```python
from build123d import *

# Parameters (mm, degrees)
SKETCH6_R                = 15
SKETCH6_R_2              = 11
BOSS_EXTRUDE2_DEPTH      = 21.3
SKETCH4_W                = 19.7
SKETCH4_H                = 3
BOSS_EXTRUDE3_REACH      = 38.107
SKETCH9_W                = 21.3
SKETCH9_H                = 9.16515139
BOSS_EXTRUDE4_START      = 0.75
SKETCH10_R               = 15
SKETCH10_R_2             = 14.25
BOSS_EXTRUDE4_DEPTH      = 0.75
CHAMFER1_SIZE            = 0.5
CHAMFER1_OF_MIRROR1_SIZE = 0.5
BOSS_EXTRUDE6_DEPTH      = 21.3
SKETCH17_W               = 18.5
SKETCH17_H               = 23.6
CUT_EXTRUDE3_DEPTH       = 2
SKETCH14_R               = 11
CUT_EXTRUDE2_DEPTH       = 31.061936082
SKETCH18_W               = 32
SKETCH18_H               = 36
BOSS_EXTRUDE7_DEPTH      = 4
SKETCH19_W               = 28.2
SKETCH19_H               = 32.35
CUT_EXTRUDE4_DEPTH       = 2
SKETCH20_W               = 6
SKETCH20_H               = 16
SKETCH20_W_2             = 8
CUT_EXTRUDE5_DEPTH       = 1
SKETCH21_W               = 1.9
SKETCH21_H               = 16
SKETCH21_H_2             = 16.00994424
CUT_EXTRUDE6_DEPTH       = 0.5
SKETCH22_W               = 18.909915591
SKETCH22_H               = 1.825
CUT_EXTRUDE7_DEPTH       = 2
FILLET1_R                = 6
FILLET2_R                = 3


# Read off the part's stored shape, not the designer's step: Boss-Extrude6
with BuildPart() as part:
    # Sketch6 → Boss-Extrude2 (new body)
    with BuildSketch(Plane(origin=(0, 0, 0), x_dir=(0, 0, -1), z_dir=(1, 0, 0))):
        Circle(SKETCH6_R)
        Circle(SKETCH6_R_2, mode=Mode.SUBTRACT)
    extrude(amount=BOSS_EXTRUDE2_DEPTH)

    # Sketch4 → Cut-Revolve1 (revolve, cut)
    with BuildSketch(Plane.XY, mode=Mode.PRIVATE) as cut_revolve1_sk:
        with Locations((10.65, -13.5)):
            Rectangle(SKETCH4_W, SKETCH4_H)
    revolve(cut_revolve1_sk.sketch.rotate(Axis((-11.602577702, 0, 0), (1, 0, 0)), 270), axis=Axis((-11.602577702, 0, 0), (1, 0, 0)), mode=Mode.SUBTRACT)

    # Sketch9 → Boss-Extrude3 (add, up to next)
    with BuildSketch(Plane.XY.offset(-10), mode=Mode.PRIVATE) as boss_extrude3_sk1:
        with Locations((10.65, 0)):
            Rectangle(SKETCH9_W, SKETCH9_H)
    boss_extrude3_tool1 = extrude(boss_extrude3_sk1.sketch, amount=-BOSS_EXTRUDE3_REACH, mode=Mode.PRIVATE) - part.part
    add(boss_extrude3_tool1.solids().sort_by_distance((10.65, 0, -10))[0])

    # Sketch10 → Boss-Extrude4 (add)
    with BuildSketch(Plane.ZY.offset(-20.5).offset(BOSS_EXTRUDE4_START)):
        Circle(SKETCH10_R)
        Circle(SKETCH10_R_2, mode=Mode.SUBTRACT)
    boss_extrude4 = extrude(amount=-BOSS_EXTRUDE4_DEPTH)

    # Chamfer1
    chamfer1_edges = [part.edges().sort_by_distance(p)[0] for p in [
        (19.75, 0, -14.25),
    ]]
    chamfer(chamfer1_edges, length=CHAMFER1_SIZE)

    # Mirror1: Boss-Extrude4 across plane
    add(boss_extrude4.mirror(Plane.ZY.offset(-10.65)))

    # Chamfer1 of Mirror1
    chamfer1_of_mirror1_edges = [part.edges().sort_by_distance(p)[0] for p in [
        (1.55, 0, -14.25),
    ]]
    chamfer(chamfer1_of_mirror1_edges, length=CHAMFER1_OF_MIRROR1_SIZE)

    # Boss-Extrude6 outline → Boss-Extrude6 (add)
    with BuildSketch(Plane.YZ):
        with BuildLine():
            Line((13.266430469, -15), (13.266430469, 15.001))
            Line((13.266430469, 15.001), (-11.733569531, 15.001))
            Line((-11.733569531, 15.001), (-11.733569531, 2.514626428))
            ThreePointArc((-11.733569531, 2.514626428), (12, 0), (-11.733569531, -2.514626428))
            Line((-11.733569531, -2.514626428), (-11.733569531, -15))
            Line((-11.733569531, -15), (13.266430469, -15))
        make_face()
    extrude(amount=BOSS_EXTRUDE6_DEPTH)

    # Sketch17 → Cut-Extrude3 (cut)
    with BuildSketch(Plane(origin=(0, 0, -15), x_dir=(-1, 0, 0), z_dir=(0, 0, -1))):
        with Locations((-10.65, 0.066430469)):
            Rectangle(SKETCH17_W, SKETCH17_H)
    extrude(amount=-CUT_EXTRUDE3_DEPTH, mode=Mode.SUBTRACT)

    # Sketch14 → Cut-Extrude2 (cut, through all)
    with BuildSketch(Plane(origin=(21.3, 0, 0), x_dir=(0, 0, -1), z_dir=(1, 0, 0))):
        Circle(SKETCH14_R)
    extrude(amount=-CUT_EXTRUDE2_DEPTH, mode=Mode.SUBTRACT)

    # Sketch18 → Boss-Extrude7 (add)
    with BuildSketch(Plane.XY.offset(15.001)):
        with Locations((10.65, 0)):
            Rectangle(SKETCH18_W, SKETCH18_H)
    extrude(amount=BOSS_EXTRUDE7_DEPTH)

    # Sketch19 → Cut-Extrude4 (cut)
    with BuildSketch(Plane.XY.offset(19.001)):
        with Locations((10.65, 0)):
            Rectangle(SKETCH19_W, SKETCH19_H)
    extrude(amount=-CUT_EXTRUDE4_DEPTH, mode=Mode.SUBTRACT)

    # Sketch20 → Cut-Extrude5 (cut)
    with BuildSketch(Plane.XY.offset(17.001)):
        with Locations((-0.45, 0)):
            Rectangle(SKETCH20_W, SKETCH20_H)
        with Locations((20.75, 0)):
            Rectangle(SKETCH20_W_2, SKETCH20_H)
    extrude(amount=-CUT_EXTRUDE5_DEPTH, mode=Mode.SUBTRACT)

    # Sketch21 → Cut-Extrude6 (cut)
    with BuildSketch(Plane.XY.offset(19.001)):
        with Locations((25.7, 0)):
            Rectangle(SKETCH21_W, SKETCH21_H)
        with Locations((-4.4, 0.459988306)):
            Rectangle(SKETCH21_W, SKETCH21_H_2)
    extrude(amount=-CUT_EXTRUDE6_DEPTH, mode=Mode.SUBTRACT)

    # Sketch22 → Cut-Extrude7 (cut)
    with BuildSketch(Plane.XY.offset(19.001)):
        with Locations((10.730756322, -17.0875)):
            Rectangle(SKETCH22_W, SKETCH22_H)
    extrude(amount=-CUT_EXTRUDE7_DEPTH, mode=Mode.SUBTRACT)

    # Fillet1
    # the kernel refuses this fillet: 6 mm, written as the material it adds along each edge
    with BuildSketch(Plane(origin=(0, -11.733569531, 15.001), x_dir=(0, -1, 0), z_dir=(1, 0, 0))) as fillet1_piece_1:
        with BuildLine():
            CenterArc((FILLET1_R, FILLET1_R), FILLET1_R, 180, 90)
            Line((0, FILLET1_R), (-FILLET1_R * 0.02, FILLET1_R))
            Line((-FILLET1_R * 0.02, FILLET1_R), (-FILLET1_R * 0.02, -FILLET1_R * 0.02))
            Line((-FILLET1_R * 0.02, -FILLET1_R * 0.02), (FILLET1_R, -FILLET1_R * 0.02))
            Line((FILLET1_R, -FILLET1_R * 0.02), (FILLET1_R, 0))
        make_face()
    extrude(amount=21.3)
    with BuildSketch(Plane(origin=(0, 13.266430469, 15.001), x_dir=(0, 1, 0), z_dir=(1, 0, 0))) as fillet1_piece_2:
        with BuildLine():
            CenterArc((6, -5.86482343), FILLET1_R, 102.185166617, 77.814833383)
            Line((0, -5.86482343), (-0.12, -5.86482343))
            Line((-0.12, -5.86482343), (-0.12, 0))
            Line((-0.12, 0), (0, 0.12))
            ThreePointArc((0, 0.12), (2.366784766, 0.12), (4.708240922, 0.117296469))
            Line((4.708240922, 0.117296469), (4.733569531, 0))
        make_face()
    extrude(amount=21.3)

    # Fillet2
    # the kernel refuses this fillet: 3 mm, written as the material it takes off along each edge
    with BuildSketch(Plane(origin=(1.4, -11.733569531, -13), x_dir=(0, -1.6111438109570978e-10, 1.0), z_dir=(1, 0, 0))) as fillet2_piece_1:
        with BuildLine():
            CenterArc((FILLET2_R, -FILLET2_R), FILLET2_R, 89.999999991, 90)
            Line((-FILLET2_R * 1.6111438107e-10, -FILLET2_R), (0, 0))
            Line((0, 0), (FILLET2_R, 0))
        make_face()
    extrude(amount=18.5, mode=Mode.SUBTRACT)
    with BuildSketch(Plane(origin=(27.685714118, -18, 17.001), x_dir=(0, 0, -1), z_dir=(-1, 0, 0))) as fillet2_piece_2_section:
        with BuildLine():
            CenterArc((FILLET2_R, -FILLET2_R), FILLET2_R, 90, 90)
            Line((0, -FILLET2_R), (0, 0))
            Line((0, 0), (FILLET2_R, 0))
        make_face()
    fillet2_piece_2 = extrude(amount=33.90991559, mode=Mode.PRIVATE)
    fillet2_piece_2 = split(fillet2_piece_2, bisect_by=Plane(origin=(22.467857059, -16.175, 16.929617158), z_dir=(0, 1, 0)), keep=Keep.TOP, mode=Mode.PRIVATE)
    fillet2_piece_2 = split(fillet2_piece_2, bisect_by=Plane(origin=(24.75, -15.883648186, 16.929617158), z_dir=(-1, 0, 0)), keep=Keep.TOP, mode=Mode.PRIVATE)
    fillet2_piece_2 = split(fillet2_piece_2, bisect_by=Plane(origin=(-3.45, -15.883648186, 16.929617158), z_dir=(1, 0, 0)), keep=Keep.TOP, mode=Mode.PRIVATE)
    add(fillet2_piece_2, mode=Mode.SUBTRACT)
    with BuildSketch(Plane(origin=(20.185714118, -18, 17.001), x_dir=(0, 0, -1), z_dir=(-1, 0, 0))) as fillet2_piece_3:
        with BuildLine():
            CenterArc((FILLET2_R, -FILLET2_R), FILLET2_R, 90, 90)
            Line((0, -FILLET2_R), (0, 0))
            Line((0, 0), (FILLET2_R, 0))
        make_face()
    extrude(amount=18.90991559, mode=Mode.SUBTRACT)


solid = part.part
```
Verification items for the finished model (mm, model axes). A direction names the side the tool comes from. Give positions to 0.01 mm unless a question says otherwise; leave off trailing zeros. Loops run counter-clockwise (first coordinate to the right, second up) from the corner with the lowest first, then second, coordinate; pieces in that order, holes last. Notation, with made-up numbers: M 60.25,-37 L 80.25,-37 A9 cw 80.25,-32 Z; hole C 31.25,55.5 d1. An arc over 180 degrees is marked long. Return JSON: item names as keys, results as strings.
1) Tool access check on faces 5 (the flat face through (21.3, 12, 0)), 6 (the flat face through (20.186, -17, 17)), 7 (the flat face through (0.8, 14, 0)). Record the directions out of +Z, -Z, +X, -X, +Y, -Y that give a thin tool (end or side, any length) a straight path to the whole face; none if there is none.
Findings:
{"face 5": "-Z, +X, +Y, -Y", "face 6": "+Z, -Y", "face 7": "none"}
2) Gauge pin test, flat ends, axial feed: P1, Ø1.4, axis at y = 14, z = 0, coming from the +X side; P2, Ø3, axis at x = -1.5, y = -3.5, coming from the +Z side; P3, Ø14, axis at x = 13, y = -5, coming from the +Z side; P4, Ø10, axis at y = -4, z = 3, coming from the +X side. Record the tip position at first contact, or that the pin passes through.
Findings:
{"P1": "stops at x = 21.3", "P2": "stops at z = 16", "P3": "stops at z = 17", "P4": "passes through"}
3) Section check D-D, the plane x = -0.5. Enter the section's corners in (y, z) (3 decimals), and give its area (3 significant figures).
Findings:
{"outline": "M -18,15.001 L 18,15.001 L 18,19.001 L 16.175,19.001 L 16.175,17.001 L 8,17.001 L 8,16.001 L -8,16.001 L -8,17.001 L -15,17.001 A3 ccw -16.175,16.761 L -16.175,19.001 L -18,19.001 Z", "area": "63.2 mm2"}
4) Section check A-A, the plane y = 0. Enter the section's corners in (x, z).
Findings:
{"outline": "M -5.35,15 L 0,15 L 0,11 L 21.3,11 L 21.3,15 L 26.65,15 L 26.65,18.5 L 24.75,18.5 L 24.75,16 L 16.75,16 L 16.75,17 L 2.55,17 L 2.55,16 L -3.45,16 L -3.45,18.5 L -5.35,18.5 Z; M 0,-15 L 1.4,-15 L 1.4,-13 L 19.9,-13 L 19.9,-15 L 21.3,-15 L 21.3,-11 L 0,-11 Z"}
5) Section check C-C, the plane x = 19. Enter the section's corners in (y, z) (3 decimals).
Findings:
{"outline": "M -17.828,15.001 L -17.734,15.001 A6 cw -11.734,9.001 L -11.734,2.515 A12 ccw -11.734,-2.515 L -11.734,-10 A3 ccw -8.734,-13 L 11.866,-13 L 11.866,-15 L 13.266,-15 L 13.266,9.136 A6 cw 18,15.001 L 18,19.001 L 16.175,19.001 L 16.175,17.001 L 8,17.001 L 8,16.001 L -8,16.001 L -8,17.001 L -15,17.001 A3 ccw Z; hole C 0,0 d22"}
6) Section check B-B, the plane z = 0. Enter the section's corners in (x, y).
Findings:
{"outline": "M 0,-15 L 1.55,-15 L 1.55,-14.75 L 1.05,-14.25 L 0.8,-14.25 L 0.8,-12 L 20.5,-12 L 20.5,-14.25 L 20.25,-14.25 L 19.75,-14.75 L 19.75,-15 L 21.3,-15 L 21.3,-11 L 0,-11 Z; M 0,11 L 21.3,11 L 21.3,15 L 19.75,15 L 19.75,14.75 L 20.25,14.25 L 20.5,14.25 L 20.5,13.27 L 0.8,13.27 L 0.8,14.25 L 1.05,14.25 L 1.55,14.75 L 1.55,15 L 0,15 Z"}
7) Mould release check, pull along Y, two halves, no side actions. Record for faces 1 (the flat face through (21, 0, 16.001)), 2 (the cylindrical face through (1, -15, 0)), 3 (the flat face through (16.75, -0.1, 16.5)), 4 (the flat face through (1.276, -17, 17)): released by +Y, released by -Y, zero draft, split by the parting line, or undercut.
Findings:
{"face 1": "undercut", "face 2": "released by -Y", "face 3": "undercut", "face 4": "zero draft"}
8) Material ranges on L1, parallel to Y at x = 5, z = 0; L2, parallel to Z at x = 9, y = 13; L3, parallel to X at y = -9.5, z = 7.5, recorded low to high. Write a range as [from, to].
Findings:
{"L1": "y = [-12, -11], [11, 13.27]", "L2": "z = [-15, 17]", "L3": "x = [0, 21.3]"}
